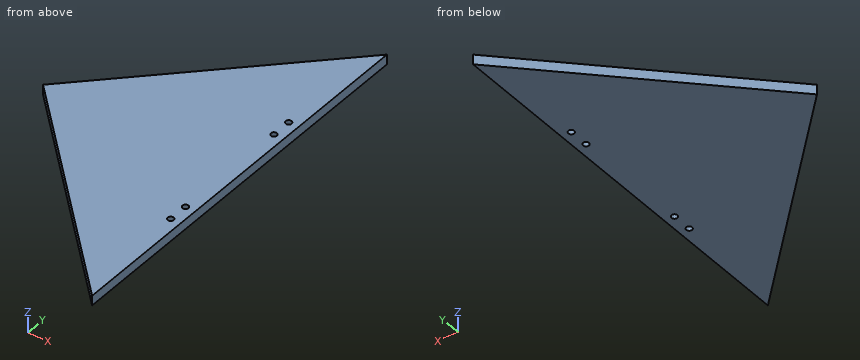
```python
from build123d import *

# Parameters (mm, degrees)
SKETCH2_R           = 1.5
BOSS_EXTRUDE1_DEPTH = 5


with BuildPart() as part:
    # Sketch2 → Boss-Extrude1 (new body)
    with BuildSketch(Plane.XY):
        Polygon((0, -100), (0, 100), (-100, 0), align=None)
        with Locations((-5, 40)):
            Circle(SKETCH2_R, mode=Mode.SUBTRACT)
        with Locations((-5, 30)):
            Circle(SKETCH2_R, mode=Mode.SUBTRACT)
        with Locations((-5, -30)):
            Circle(SKETCH2_R, mode=Mode.SUBTRACT)
        with Locations((-5, -40)):
            Circle(SKETCH2_R, mode=Mode.SUBTRACT)
    extrude(amount=BOSS_EXTRUDE1_DEPTH)


solid = part.part
```
Work out the finished part from the listing and answer in its coordinate system (mm). Round coordinates to 2 decimals unless told otherwise and drop trailing zeros. Loops run counter-clockwise (first coordinate to the right, second up) from the corner with the lowest first, then second, coordinate; pieces in that order, holes last.
(1) The part is cut by section B-B, the plane y = -83.5. Give the vertices of the cut face in (x, z), and give its area (3 significant figures).
Computed values:
outline: (-16.5, 0) - (0, 0) - (0, 5) - (-16.5, 5) - close
area: 82.5 mm2
(2) The part is cut by section C-C, the plane x = -86.5. Give the vertices of the cut face in (y, z).
Computed values:
outline: (-13.5, 0) - (13.5, 0) - (13.5, 5) - (-13.5, 5) - close
(3) The part is cut by section A-A, the plane z = 1.5. Give the vertices of the cut face in (x, y).
Computed values:
outline: (-100, 0) - (0, -100) - (0, 100) - close; hole circle Ø3 at (-5, -40); hole circle Ø3 at (-5, -30); hole circle Ø3 at (-5, 30); hole circle Ø3 at (-5, 40)
(4) Each of these flat-tipped pins is pushed along its axis until it touches: P1, Ø2.5, axis at x = -5, y = -40, coming from the +Z side; P2, Ø3, axis at x = -63, z = 1, coming from the -Y side. Where does it stop, or does it pass through?
Computed values:
P1: passes through
P2: stops at y = -38.5
(5) Find the intervals of material crossed by L1, parallel to Y at x = -5, z = 2.7; L2, parallel to X at y = 50.5, z = 0.4; L3, parallel to Y at x = -83, z = 2.8, in increasing order.
Computed values:
L1: y = -95 to -41.5, -38.5 to -31.5, -28.5 to 28.5, 31.5 to 38.5, 41.5 to 95
L2: x = -49.5 to 0
L3: y = -17 to 17
